The listing builds one solid part. Answer for the finished solid, in the listing's coordinates (mm). Give positions to 0.01 mm unless a question says otherwise; leave off trailing zeros. Loops run counter-clockwise (first coordinate to the right, second up) from the corner with the lowest first, then second, coordinate; pieces in that order, holes last. Notation, with made-up numbers: (75.5, 8.5) - (120.5, 8.5) arc R15 cw to (120.5, 26.5) - close; hole circle Ø6 at (-12.5, 84.5). An arc over 180 degrees is marked (long way). Write each question's results on one line, items separated by ' | '.
from build123d import *

# Parameters (mm, degrees)
BOSS_EXTRUDE1_DEPTH = 4
SKETCH2_R           = 1.6
SKETCH2_W           = 16
SKETCH2_H           = 5
CUT_EXTRUDE1_DEPTH  = 108.154094649


with BuildPart() as part:
    # Sketch1 → Boss-Extrude1 (new body)
    with BuildSketch(Plane.XY):
        Polygon((-95, 17), (-100, 17), (-100, 21), (-105, 21), (-105, 12.500446192), (-74.214666133, -1), (-74.214666133, -12.643441465), (-62, -18), (-2, -18), (-2, -6), (2, -6), (2, -18), (62, -18), (74.214666133, -12.643441465), (74.214666133, -1), (105, 12.500446192), (105, 21), (100, 21), (100, 17), (95, 17), (90.439360532, 15), (2, 15), (2, 9), (-2, 9), (-2, 15), (-90.439360532, 15), align=None)
    extrude(amount=BOSS_EXTRUDE1_DEPTH)

    # Sketch2 → Cut-Extrude1 (cut, through all)
    with BuildSketch(Plane.XY.offset(4)):
        with Locations((62, 12)):
            Circle(SKETCH2_R)
        with Locations((62, -7.5)):
            Rectangle(SKETCH2_W, SKETCH2_H)
    cut_extrude1 = extrude(amount=-CUT_EXTRUDE1_DEPTH, mode=Mode.SUBTRACT)

    # Mirror1: Cut-Extrude1 across plane
    add(cut_extrude1.mirror(Plane(origin=(0, 0, 0), x_dir=(0, 0, 1), z_dir=(1, 0, 0))), mode=Mode.SUBTRACT)


solid = part.part
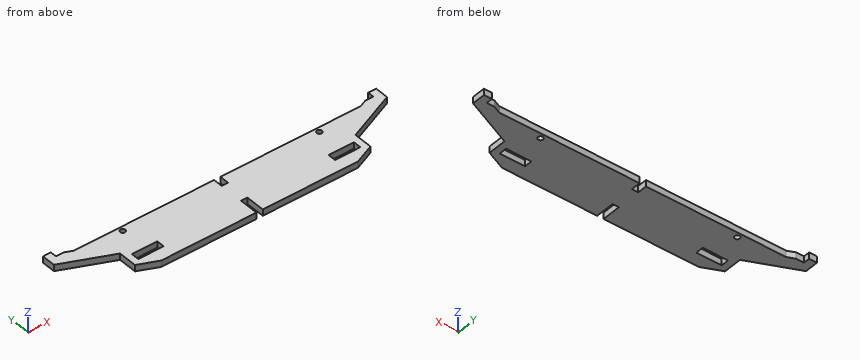
Item 1: A cutting plane is placed at A-A, the plane z = 3.2. Count the separate pieces of the cut face and the enclosed holes in it, plus the area to 3 significant figures.
Values found:
separate pieces: 1 | enclosed holes: 4 | area: 5,240 mm²
Item 2: Find the intervals of material crossed by line 1 along Y through (x, z) = (62, 1.75); line 2 along X through (y, z) = (-5.5, 2.95); line 3 along X through (y, z) = (-7.5, 2.2), in increasing order. Write a range as [from, to].
Values found:
line 1: y = [-18, -10], [-5, 10.4], [13.6, 15] | line 2: x = [-74.21, -70], [-54, 54], [70, 74.21] | line 3: x = [-74.21, -70], [-54, -2], [2, 54], [70, 74.21]
Item 3: A cutting plane is placed at C-C, the plane x = -72. Determine the outline of the cut face in (y, z), plus the area to 3 significant figures.
Values found:
outline: (-13.61, 0) - (15, 0) - (15, 4) - (-13.61, 4) - close | area: 114 mm²
Item 4: Flat-ended cylindrical pins translate along their axes: P1, Ø12, axis at x = -60.5, y = 1, coming from the -Z side; P2, Ø1.2, axis at y = -7, z = 2.5, coming from the -X side; P3, Ø1.2, axis at x = 27, z = 2.5, coming from the +Y side; P4, Ø1.2, axis at y = -7, z = 2.5, coming from the +X side. Find the tip coordinate at first contact, or state that the pin passes through.
Values found:
P1: stops at z = 0 | P2: stops at x = -74.21 | P3: stops at y = 15 | P4: stops at x = 74.21
Item 5: A cutting plane is placed at B-B, the plane x = 5.5. Determine the outline of the cut face in (y, z).
Values found:
outline: (-18, 0) - (15, 0) - (15, 4) - (-18, 4) - close
